The model under review builds one solid part; all positions refer to its coordinate system, in mm. Face numbers are marked on the shaded views. A direction names the side the tool comes from. Coordinates: 2 decimals unless noted, no trailing zeros. Write each loop counter-clockwise with the first axis right and the second up, starting at its lowest first coordinate (ties: lowest second). Pieces come first, ordered by that corner, then holes.
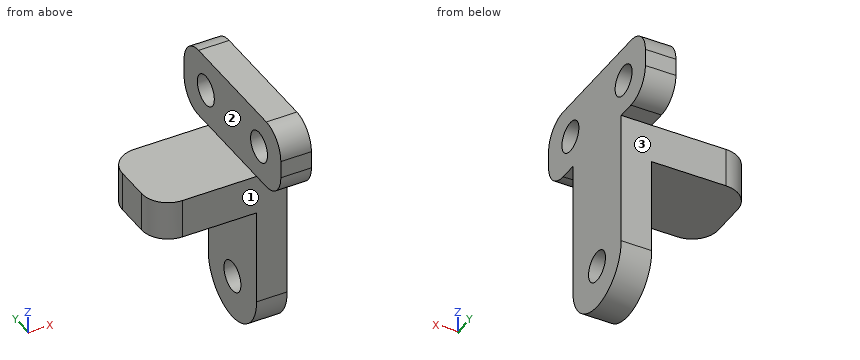
```python
from build123d import *

# Parameters (mm, degrees)
SKETCH023_R              = 1.75
PAD024_DEPTH             = 40
PAD025_DEPTH             = 70
FILLET011_R              = 3
CLONE136_PLACEMENT_ANGLE = 180


with BuildPart() as pad024:
    # Sketch023 → Pad024 (new body)
    with BuildSketch(Plane(origin=(-50, 0, 0), x_dir=(0, -1, 0), z_dir=(-1, 0, 0))):
        with BuildLine():
            ThreePointArc((-5, 18), (1e-05, 13), (5, 18.000021))
            Line((5, 33.500021), (5, 18.000021))
            Line((10, 33.500021), (5, 33.500021))
            Line((10, 41.5), (10, 33.500021))
            Line((-10, 41.5), (10, 41.5))
            Line((-10, 33.5), (-10, 41.5))
            Line((-5, 33.5), (-10, 33.5))
            Line((-5, 18), (-5, 33.5))
        make_face()
        with Locations((-5.5, 37.5)):
            Circle(SKETCH023_R, mode=Mode.SUBTRACT)
        with Locations((5.5, 37.5)):
            Circle(SKETCH023_R, mode=Mode.SUBTRACT)
        with Locations((0, 18)):
            Circle(SKETCH023_R, mode=Mode.SUBTRACT)
    extrude(amount=-PAD024_DEPTH)


with BuildPart() as clone_of_support003:
    # Sketch022 → Pad025 (new body)
    with BuildSketch(Plane.XZ.offset(40)):
        Polygon((-31.5, 12), (-35, 12), (-35, 53.5), (-31.5, 53.5), (-31.5, 33.5), (-20, 33.5), (-20, 29), (-31.5, 29), align=None)
    extrude(amount=-PAD025_DEPTH)

    # Common001: intersect Pad024
    add(pad024.part, mode=Mode.INTERSECT)

    # Fillet011
    fillet011_edges = [clone_of_support003.edges().sort_by_distance(p)[0] for p in [
        (-20, -5, 31.25),
        (-20, 5, 31.25),
        (-33.25, -10, 33.500021),
        (-33.25, 10, 33.5),
        (-33.25, -10, 41.5),
        (-33.25, 10, 41.5),
    ]]
    fillet(fillet011_edges, radius=FILLET011_R)


with BuildPart() as clone_of_support003_1:
    # Clone136 placement: moved
    add(clone_of_support003.part.rotate(Axis((0, 0, 0), (0, 0, 1)), CLONE136_PLACEMENT_ANGLE))


solid = clone_of_support003_1.part
```
Item 1: Machinability: for the marked faces 1, 2 and 3, which of the approach directions +Z, -Z, +X, -X, +Y, -Y give a long, thin tool a straight path to every point of the face, cutting with its end or side? Answer none if there is none.
Solved:
face 1: -Z, +X, -X, -Y
face 2: +Z, -X, +Y, -Y
face 3: -Z, +X, -X, +Y
Item 2: To check wall thickness, follow line 1 along Y through (x, z) = (34, 20.75); line 2 along Z through (x, y) = (21.5, -2.25); line 3 along X through (y, z) = (-5, 35.5). State the ranges of each line that lie inside material, in increasing order.
Solved:
line 1: y = -5 to 5
line 2: z = 29 to 33.5
line 3: x = 31.5 to 35
Item 3: For pin 1 (3 mm diameter, centred on y = -3, z = 19, fed in from -X); pin 2 (0.6 mm diameter, centred on x = 32.5, y = -6.5, fed in from -Z); pin 3 (2 mm diameter, centred on x = 21.5, y = -3.5, fed in from -Z), all flat-tipped, find the tip position at first contact; note any pin that passes through.
Solved:
pin 1: stops at x = 31.5
pin 2: stops at z = 33.5
pin 3: stops at z = 29
Item 4: Take a section at A-A, the plane z = 37.5. Write out the cut boundary in (x, y).
Solved:
outline: (31.5, -10) - (35, -10) - (35, -7.25) - (31.5, -7.25) - close; (31.5, -3.75) - (35, -3.75) - (35, 3.75) - (31.5, 3.75) - close; (31.5, 7.25) - (35, 7.25) - (35, 10) - (31.5, 10) - close
Item 5: Take a section at C-C, the plane x = 24. Write out the cut boundary in (y, z).
Solved:
outline: (-5, 29) - (5, 29) - (5, 33.5) - (-5, 33.5) - close
Item 6: Take a section at B-B, the plane y = 5.5. Write out the cut boundary in (x, z).
Solved:
outline: (31.5, 33.5) - (35, 33.5) - (35, 35.75) - (31.5, 35.75) - close; (31.5, 39.25) - (35, 39.25) - (35, 41.5) - (31.5, 41.5) - close
Item 7: Take a section at D-D, the plane z = 29.75. Write out the cut boundary in (x, y), plus the area to 3 significant figures.
Solved:
outline: (20, -2) arc R3 ccw to (23, -5) - (35, -5) - (35, 5) - (23, 5) arc R3 ccw to (20, 2) - close
area: 146 mm2
